The listing builds one solid part. Answer for the finished solid, in the listing's coordinates (mm). Face numbers are marked on the shaded views. Give positions to 0.01 mm unless a question says otherwise; leave off trailing zeros. Loops run counter-clockwise (first coordinate to the right, second up) from the corner with the lowest first, then second, coordinate; pieces in that order, holes last. Notation, with made-up numbers: M 29.25,79.5 L 51.25,79.5 A20 ccw 51.25,100.5 Z; hole C 24,-14 d9. An arc over 180 degrees is marked long. Use one line per item in the form item = value. Start each with the question number.
1. Straight lines are drawn through the part: line 1 (Z direction, x = -1, y = 69); line 2 (Y direction, x = 2, z = -6); line 3 (X direction, y = -19, z = 23). For each, find the intervals that lie inside material, in ascending order. Write a range as from..to.
2. Each of these flat-tipped pins is pushed along its axis until it touches: pin 1 Ø1.5 at (y, z) = (12, 27.5) entering from -X; pin 2 Ø10 at (x, y) = (18, 55) entering from -Z; pin 3 Ø10 at (x, z) = (23.5, 26.5) entering from +Y. Where does it stop, or does it pass through?
3. The part is cut by section C-C (y = 7.5). Write down the section's boundary in (x, z) (3 decimals).
4. The mould has two halves that part along Y. Classify the marked faces 1, 2 and 3: released by +Y, released by -Y, zero draft, split by the parting line, or undercut.
5. The part is cut by section B-B (x = 0). Write down the section's boundary in (y, z) (3 decimals).
6. The part is cut by section D-D (x = -24). Write down the section's boundary in (y, z) (3 decimals), and give its area (3 significant figures).
7. The part is cut by section A-A (z = 0). Write down the section's boundary in (x, y) (3 decimals), and give its area (3 significant figures).
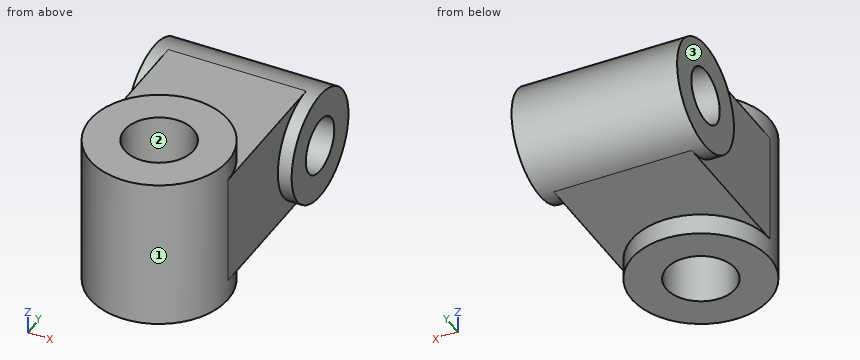
Autodesk Inventor part; units mm, degrees
ref_plane "YZ Plane" through (0, 0, 0) normal (1, 0, 0) x (0, 1, 0)
ref_plane "XZ Plane" through (0, 0, 0) normal (0, 1, 0) x (-1, 0, 0)
ref_plane "XY Plane" through (0, 0, 0) normal (0, 0, 1) x (1, 0, 0)
sketch "Sketch1" plane through (0, 0, 0) normal (0, 0, 1) x (1, 0, 0)
  circle A0 centre (0, 0) radius 31.75
  circle A1 centre (0, 0) radius 15.875
  dimension "d0" = 63.5
  dimension "d1" = 31.75
extrude "Extrusion1" add sketch "Sketch1" along normal mid plane 69.85
sketch "Sketch2" plane through (0, 0, 0) normal (1, 0, 0) x (0, 1, 0)
  line L0 (0, 0) -> (69.85, 0) construction
  circle A0 centre (69.85, 0) radius 25.4
  circle A1 centre (69.85, 0) radius 12.7
  dimension "d4" = 69.85
  dimension "d5" = 50.8
  dimension "d6" = 25.4
extrude "Extrusion2" add sketch "Sketch2" along normal mid plane 76.2
sketch "Sketch3" plane through (0, 0, 0) normal (0, 1, 0) x (-1, 0, 0)
  line L0 (-31.75, -34.925) -> (31.75, -34.925)
  line L1 (31.75, 34.925) -> (-31.75, 34.925)
  line L2 (-31.75, -34.925) -> (-31.75, 34.925)
  line L3 (31.75, -34.925) -> (31.75, 34.925)
  line L4 (38.1, -25.4) -> (38.1, 25.4)
  line L5 (-38.1, 25.4) -> (-38.1, -25.4)
  line L6 (38.1, 25.4) -> (-38.1, 25.4)
  line L7 (38.1, -25.4) -> (-38.1, -25.4)
  line L8 (31.75, 25.4) -> (-31.75, 25.4)
  line L9 (-31.75, -25.4) -> (-31.75, 25.4)
  line L10 (-31.75, -25.4) -> (31.75, -25.4)
  line L11 (31.75, 25.4) -> (31.75, -25.4)
  point P0 (0, 0)
extrude "Extrusion3" add sketch "Sketch3" along normal up to surface contours L2 L6 L3 L7
sketch "Sketch4" plane through (0, 0, 34.925) normal (0, 0, 1) x (1, 0, 0)
  circle A0 centre (0, 0) radius 15.875
extrude "Extrusion4" cut sketch "Sketch4" against normal through all
properties part number "TubeSpacer"
Derived:
q1.line_1 = -25.4..-12.67, 12.67..25.4
q1.line_2 = -31.69..-15.75, 15.75..58.66, 81.04..94.53
q1.line_3 = -25.44..25.44
q2.pin_1 = -29.69
q2.pin_2 = -25.4
q2.pin_3 = 83.37
q3.outline = M -31.75,-25.4 L -30.851,-25.4 L -30.851,-34.925 L -13.992,-34.925 L -13.992,34.925 L -30.851,34.925 L -30.851,25.4 L -31.75,25.4 Z; M 13.992,-34.925 L 30.851,-34.925 L 30.851,-25.4 L 31.75,-25.4 L 31.75,25.4 L 30.851,25.4 L 30.851,34.925 L 13.992,34.925 Z
q4.face_1 = split by the parting line
q4.face_2 = undercut
q4.face_3 = zero draft
q5.outline = M -31.75,-34.925 L -15.875,-34.925 L -15.875,34.925 L -31.75,34.925 Z; M 15.875,-34.925 L 31.75,-34.925 L 31.75,-25.4 L 69.85,-25.4 A25.4 ccw 69.85,25.4 L 31.75,25.4 L 31.75,34.925 L 15.875,34.925 Z; hole C 69.85,0 d25.4
q6.outline = M -20.786,-34.925 L 20.786,-34.925 L 20.786,-25.4 L 69.85,-25.4 A25.4 ccw 69.85,25.4 L 20.786,25.4 L 20.786,34.925 L -20.786,34.925 Z; hole C 69.85,0 d25.4
q6.area = 5,900 mm2
q7.outline = M -38.1,44.45 L -31.75,44.45 L -31.75,0 A31.75 ccw 31.75,0 L 31.75,44.45 L 38.1,44.45 L 38.1,57.15 L -38.1,57.15 Z; M -38.1,82.55 L 38.1,82.55 L 38.1,95.25 L -38.1,95.25 Z; hole C 0,0 d31.75
q7.area = 5,550 mm2
